from build123d import *

# Parameters (mm, degrees)
F0_W     = 16.238193959
F0_H     = 11.2191159278
F0_W_2   = 11.5143544972
F0_W_3   = 16.459621489
F0_H_2   = 20.3715497628
F0_H_3   = 11.5143535659
F0_W_4   = 15.942953527
F1_DEPTH = 8.128


with BuildPart() as f1:
    # F0 (on Top) → F1 (new body)
    with BuildSketch(Plane.XY):
        with Locations((-36.0930729657, 18.0834410712)):
            Rectangle(F0_W, F0_H)
        with Locations((-22.2167987376, 18.0834410712)):
            Rectangle(F0_W_2, F0_H)
        with Locations((-8.2298107445, 18.0834410712)):
            Rectangle(F0_W_3, F0_H)
        with Locations((-22.2167987376, 2.2881082259)):
            Rectangle(F0_W_2, F0_H_2)
        with Locations((-22.2167987376, -13.6548434384)):
            Rectangle(F0_W_2, F0_H_3)
        with Locations((-35.9454527497, -13.6548434384)):
            Rectangle(F0_W_4, F0_H_3)
    extrude(amount=F1_DEPTH)


solid = f1.part
The model under review builds one solid part; all positions refer to its coordinate system, in mm. A direction names the side the tool comes from. Give positions to 0.01 mm unless a question says otherwise; leave off trailing zeros. Loops run counter-clockwise (first coordinate to the right, second up) from the corner with the lowest first, then second, coordinate; pieces in that order, holes last. Notation, with made-up numbers: (84.25, -15.5) -> (136.25, -15.5) arc R13 ccw to (136.25, -9.5) -> close; hole circle Ø8 at (37, 28). An arc over 180 degrees is marked (long way). Write each question's results on one line, items separated by ' | '.
1) For line 1 along Y through (x, z) = (-28.5, 0.75); line 2 along X through (y, z) = (7.5, 2); line 3 along Y through (x, z) = (-15.5, 1), list the stretches that pass through material, from the lowest coordinate up. Write a range as from..to.
Conclusion:
line 1: y = -19.41..-7.9, 12.47..23.69 | line 2: x = -27.97..-16.46 | line 3: y = 12.47..23.69
2) Draft analysis for pull direction Y (two halves, no side actions). For faces 1 (the face through (-43.917, -14, 4)), 2 (the face through (-8, 12.474, 4)), 3 (the face through (-27.974, 2, 4)), state which applies: pulls with the +Y half, pulls with the -Y half, needs draft (parallel to the pull), parting line crosses it, or undercut.
Conclusion:
face 1: needs draft | face 2: pulls with the -Y half | face 3: undercut
3) Take a section at A-A, the plane x = -32. Give the boundary of the cut face in (y, z), plus the area to 3 significant figures.
Conclusion:
outline: (-19.41, 0) -> (-7.9, 0) -> (-7.9, 8.13) -> (-19.41, 8.13) -> close; (12.47, 0) -> (23.69, 0) -> (23.69, 8.13) -> (12.47, 8.13) -> close | area: 185 mm^2
4) Take a section at B-B, the plane z = 5.5. Give the boundary of the cut face in (x, y), plus the area to 3 significant figures.
Conclusion:
outline: (-44.21, 12.47) -> (-27.97, 12.47) -> (-27.97, -7.9) -> (-43.92, -7.9) -> (-43.92, -19.41) -> (-16.46, -19.41) -> (-16.46, 12.47) -> (0, 12.47) -> (0, 23.69) -> (-44.21, 23.69) -> close | area: 1,050 mm^2
5) Tool access review of faces 4 (the face through (-36, 12.474, 4)), 5 (the face through (-22, 23.693, 4)), 6 (the face through (-16.46, -4, 4)): name each direction out of +Z, -Z, +X, -X, +Y, -Y from which nothing blocks a thin tool from reaching the whole face with its end or side.
Conclusion:
face 4: +Z, -Z, -X | face 5: +Z, -Z, +X, -X, +Y | face 6: +Z, -Z, +X, -Y
6) Take a section at C-C, the plane y = 4.5. Give the boundary of the cut face in (x, z), plus the area to 3 significant figures.
Conclusion:
outline: (-27.97, 0) -> (-16.46, 0) -> (-16.46, 8.13) -> (-27.97, 8.13) -> close | area: 93.6 mm^2
7) Insertion check: pin 1 Ø2.5 at (x, z) = (-7.5, 3) entering from -Y; pin 2 Ø4 at (y, z) = (-14, 4) entering from -X; pin 3 Ø1 at (y, z) = (0, 7) entering from -X. Each pin has a flat end and moves straight along its axis. Give the tip position at first contact, or say it passes through.
Conclusion:
pin 1: stops at y = 12.47 | pin 2: stops at x = -43.92 | pin 3: stops at x = -27.97
